Here's the drawing with two shaded views (mm, measured from the low corner). I have some questions. A direction names the side the tool comes from. Give positions to 0.01 mm unless a question says otherwise; leave off trailing zeros. Write each loop counter-clockwise with the first axis right and the second up, starting at its lowest first coordinate (ties: lowest second). Pieces come first, ordered by that corner, then holes. Notation, with made-up numbers: (4, 45) -> (24, 45) arc R15 ccw to (24, 54) -> close; hole circle Ø3 at (83, 81.25). An arc over 180 degrees is marked (long way). Put each result on its own line as item: value. Start each with the question number.
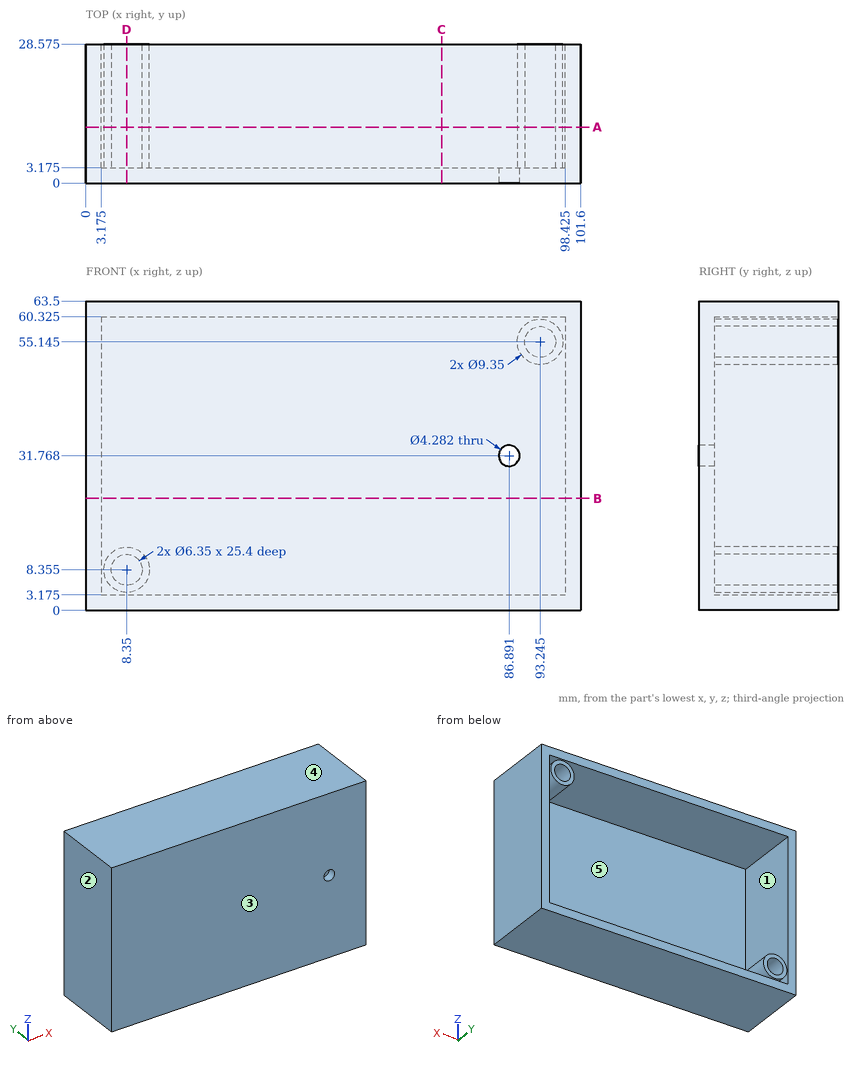
1) Which directions (+Z, -Z, +X, -X, +Y, -Y) give clear straight access to the entire face, cutting with the end or side of a thin tool? Please do the marked faces 4 and 5.
2) I need wall thicknesses on probe 1 along X at (y, z) = (13.5, 55) (1 decimal); probe 2 along Z at (x, y) = (8.35, 12.75) (1 decimal); probe 3 along X at (y, z) = (23.75, 41) (1 decimal). Which ranges of each line are inside material? Lowest first, please.
3) I want a section at D-D, the plane x = 8.35. Write out the boundary of the cut face in (y, z) (1 decimal), and give its area (3 significant figures).
4) I want a section at B-B, the plane z = 23. Write out the boundary of the cut face in (x, y) (1 decimal), and give its area (3 significant figures).
5) I'm going to push a flat-ended pin straight in: pin 1 Ø3 at (x, z) = (9.5, 8.5) entering from +Y (3 decimals). Where does the tip first touch, or does it pass through?
6) I want a section at C-C, the plane x = 73. Write out the boundary of the cut face in (y, z) (1 decimal).
7) I want a section at A-A, the plane y = 11.5. State how many separate pieces and enclosed holes the cut face has, and give its area (3 significant figures).
8) Thinking about a two-plate mould opening in X: for the marked faces 1, 2 and 3, which applies, released by +X, released by -X, zero draft, split by the parting line, or undercut?
Established:
1. face 4: +Z, +X, -X, +Y, -Y
1. face 5: +Y
2. probe 1: x = 0 to 3.2, 88.6 to 90.1, 96.4 to 97.9, 98.4 to 101.6
2. probe 2: z = 0 to 3.2, 3.7 to 5.2, 11.5 to 13, 60.3 to 63.5
2. probe 3: x = 0 to 3.2, 98.4 to 101.6
3. outline: (0, 0) -> (28.6, 0) -> (28.6, 3.2) -> (3.2, 3.2) -> (3.2, 3.7) -> (28.6, 3.7) -> (28.6, 5.2) -> (3.2, 5.2) -> (3.2, 11.5) -> (28.6, 11.5) -> (28.6, 13) -> (3.2, 13) -> (3.2, 60.3) -> (28.6, 60.3) -> (28.6, 63.5) -> (0, 63.5) -> close
3. area: 439 mm2
4. outline: (0, 0) -> (101.6, 0) -> (101.6, 28.6) -> (98.4, 28.6) -> (98.4, 3.2) -> (3.2, 3.2) -> (3.2, 28.6) -> (0, 28.6) -> close
4. area: 484 mm2
5. pin 1: stops at y = 3.175
6. outline: (0, 0) -> (28.6, 0) -> (28.6, 3.2) -> (3.2, 3.2) -> (3.2, 60.3) -> (28.6, 60.3) -> (28.6, 63.5) -> (0, 63.5) -> close
7. separate pieces: 3
7. enclosed holes: 3
7. area: 1,080 mm2
8. face 1: undercut
8. face 2: released by -X
8. face 3: zero draft
